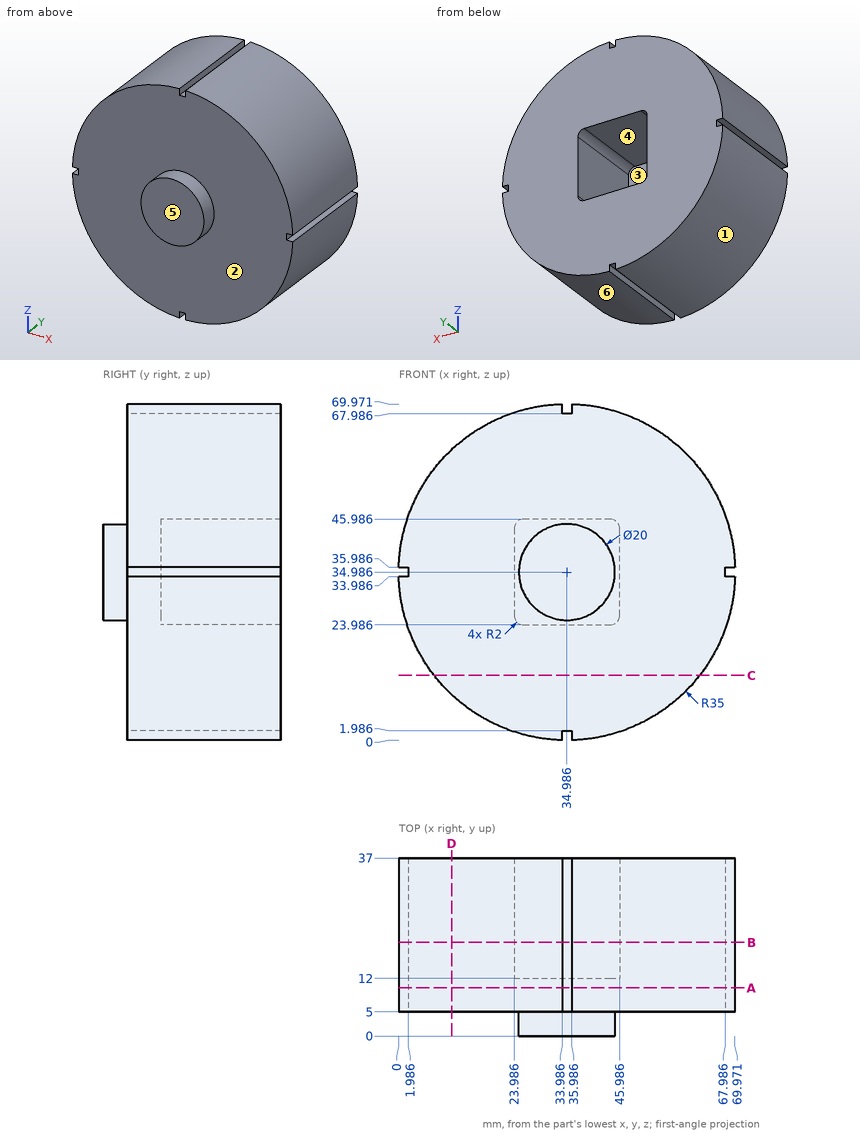
Part print with two shaded views. Sizes in mm from the minimum x, y, z corner. A direction names the side the tool comes from. Coordinates: 2 decimals unless noted, no trailing zeros. Write each loop counter-clockwise with the first axis right and the second up, starting at its lowest first coordinate (ties: lowest second). Pieces come first, ordered by that corner, then holes. Notation, with made-up numbers: (-16.75, 14.25) - (21.25, 14.25) arc R19 ccw to (21.25, 27.25) - close; hole circle Ø8 at (25.5, 77). An arc over 180 degrees is marked (long way). Use a Markdown table: item, result. Add a question column.
Item 1: Band-saw the part on B-B, the plane y = 19.5. Write the cut outline in (x, z) (1 decimal), and give its area (3 significant figures).
Item 2: Two-plate mould, pull along X, no slides. Class the marked faces 4, 5 and 6: pulls with the +X half, pulls with the -X half, needs draft (parallel to the pull), parting line crosses it, or undercut.
Item 3: 3-axis set-ups, long thin cutter, end or side, ignore diameter. For the marked faces 1, 2 and 3: which of +Z, -Z, +X, -X, +Y, -Y reach the whole face in a straight line?
Item 4: Drop flat-ended pins along their axis: pin 1 (1 mm diameter, centred on x = 35, y = 19, fed in from +Z); pin 2 (6 mm diameter, centred on y = 18.5, z = 59, fed in from +X) (1 decimal); pin 3 (8 mm diameter, centred on x = 10, y = 27, fed in from -Z) (1 decimal); pin 4 (17.5 mm diameter, centred on x = 30.5, z = 33.5, fed in from +Y). Give the stop position or say it passes through.
Item 5: Band-saw the part on D-D, the plane x = 11. Write the cut outline in (y, z) (1 decimal), and give its area (3 significant figures).
Item 6: Drill centre lines: line 1 along X through (y, z) = (31.5, 35) (1 decimal); line 2 along Y through (x, z) = (12, 61); line 3 along Y through (x, z) = (45, 45). Where is each one in solid material? Low to high.
Item 7: Band-saw the part on C-C, the plane z = 13.5. Write the cut outline in (x, y) (1 decimal).
Item 8: Band-saw the part on A-A, the plane y = 10. Write the cut outline in (x, z) (1 decimal), and give its area (3 significant figures).
A:
| question | item | result |
|---|---|---|
| 1 | outline | (0, 34) arc R35 ccw to (34, 0) - (34, 2) - (36, 2) - (36, 0) arc R35 ccw to (70, 34) - (68, 34) - (68, 36) - (70, 36) arc R35 ccw to (36, 70) - (36, 68) - (34, 68) - (34, 70) arc R35 ccw to (0, 36) - (2, 36) - (2, 34) - close; hole (24, 26) arc R2 ccw to (26, 24) - (44, 24) arc R2 ccw to (46, 26) - (46, 44) arc R2 ccw to (44, 46) - (26, 46) arc R2 ccw to (24, 44) - close |
| 1 | area | 3,350 mm² |
| 2 | face 4 | undercut |
| 2 | face 5 | needs draft |
| 2 | face 6 | pulls with the +X half |
| 3 | face 1 | -Z, -X, +Y, -Y |
| 3 | face 2 | -Y |
| 3 | face 3 | +Y |
| 4 | pin 1 | stops at z = 67.99 |
| 4 | pin 2 | stops at x = 63 |
| 4 | pin 3 | stops at z = 7 |
| 4 | pin 4 | stops at y = 37 |
| 5 | outline | (5, 9.5) - (37, 9.5) - (37, 60.5) - (5, 60.5) - close |
| 5 | area | 1,630 mm² |
| 6 | line 1 | x = 2 to 24, 46 to 68 |
| 6 | line 2 | y = 5 to 37 |
| 6 | line 3 | y = 5 to 12 |
| 7 | outline | (7.4, 5) - (62.6, 5) - (62.6, 37) - (7.4, 37) - close |
| 8 | outline | (0, 34) arc R35 ccw to (34, 0) - (34, 2) - (36, 2) - (36, 0) arc R35 ccw to (70, 34) - (68, 34) - (68, 36) - (70, 36) arc R35 ccw to (36, 70) - (36, 68) - (34, 68) - (34, 70) arc R35 ccw to (0, 36) - (2, 36) - (2, 34) - close |
| 8 | area | 3,830 mm² |
